```python
from build123d import *

# Parameters (mm, degrees)
SKETCH1_R                                           = 60.625
SKETCH1_R_2                                         = 45
BOSS_EXTRUDE1_DEPTH                                 = 4
SKETCH2_R                                           = 49
SKETCH2_R_2                                         = 45
BOSS_EXTRUDE2_DEPTH                                 = 52
SKETCH4_W                                           = 13.25
SKETCH4_H                                           = 8
SKETCH4_W_2                                         = 8
SKETCH4_H_2                                         = 38
BOSS_EXTRUDE4_DEPTH                                 = 13
BOSS_EXTRUDE5_DEPTH                                 = 4
SKETCH7_R                                           = 1.3
CUT_EXTRUDE4_DEPTH                                  = 7.2
SKETCH9_W                                           = 10
SKETCH9_H                                           = 24
CUT_EXTRUDE7_DEPTH                                  = 8
CUT_EXTRUDE8_REACH                                  = 111.625
SKETCH11_R                                          = 5
CUT_EXTRUDE9_DEPTH                                  = 5.0000001
CSK_FOR_M3_COUNTERSUNK_FLAT_HEAD_SCREW1_D           = 3.4
CSK_FOR_M3_COUNTERSUNK_FLAT_HEAD_SCREW1_DEPTH       = 4
CSK_FOR_M3_COUNTERSUNK_FLAT_HEAD_SCREW1_CSINK_D     = 6.3
CSK_FOR_M3_COUNTERSUNK_FLAT_HEAD_SCREW1_CSINK_ANGLE = 90
SKETCH18_W                                          = 98
SKETCH18_H                                          = 7
CUT_EXTRUDE10_DEPTH                                 = 61.625
CUT_EXTRUDE10_DEPTH_BACK                            = 61.625


with BuildPart() as part:
    # Sketch1 → Boss-Extrude1 (new body)
    with BuildSketch(Plane(origin=(0, 0, 0), x_dir=(1, 0, 0), z_dir=(0, 1, 0))):
        Circle(SKETCH1_R)
        Circle(SKETCH1_R_2, mode=Mode.SUBTRACT)
    extrude(amount=BOSS_EXTRUDE1_DEPTH)

    # Sketch2 → Boss-Extrude2 (add)
    with BuildSketch(Plane(origin=(0, 4, 0), x_dir=(1, 0, 0), z_dir=(0, 1, 0))):
        Circle(SKETCH2_R)
        Circle(SKETCH2_R_2, mode=Mode.SUBTRACT)
    extrude(amount=BOSS_EXTRUDE2_DEPTH)

    # Sketch4 → Boss-Extrude4 (add, symmetric)
    with BuildSketch(Plane.XY):
        with Locations((-38.375, 34)):
            Rectangle(SKETCH4_W, SKETCH4_H)
        Polygon((-31.75, 30), (-45, 30), (-45, 16.75), align=None)
        with Locations((15.25, 19)):
            Rectangle(SKETCH4_W_2, SKETCH4_H_2)
    extrude(amount=BOSS_EXTRUDE4_DEPTH, both=True)

    # Sketch5 → Boss-Extrude5 (add)
    with BuildSketch(Plane.XZ):
        with BuildLine():
            Line((11.25, 13), (29.067400866, 34.352382842))
            ThreePointArc((29.067400866, 34.352382842), (45, 0), (29.067400866, -34.352382842))
            Line((29.067400866, -34.352382842), (11.25, -13))
            Line((11.25, -13), (11.25, 13))
        make_face()
    extrude(amount=-BOSS_EXTRUDE5_DEPTH)

    # Sketch7 → Cut-Extrude4 (cut)
    with BuildSketch(Plane(origin=(0, 38, 0), x_dir=(1, 0, 0), z_dir=(0, 1, 0))):
        with Locations((-34.25, 5)):
            Circle(SKETCH7_R)
        with Locations((-34.25, -5)):
            Circle(SKETCH7_R)
        with Locations((13.75, 5)):
            Circle(SKETCH7_R)
        with Locations((13.75, -5)):
            Circle(SKETCH7_R)
    extrude(amount=-CUT_EXTRUDE4_DEPTH, mode=Mode.SUBTRACT)

    # Sketch9 → Cut-Extrude7 (cut)
    with BuildSketch(Plane.ZY.offset(-11.25)):
        with Locations((0, 17)):
            Rectangle(SKETCH9_W, SKETCH9_H)
    extrude(amount=-CUT_EXTRUDE7_DEPTH, mode=Mode.SUBTRACT)

    # Sketch11 → Cut-Extrude8 (cut, up to next)
    with BuildSketch(Plane(origin=(49, 0, 0), x_dir=(0, 0, -1), z_dir=(1, 0, 0)), mode=Mode.PRIVATE) as cut_extrude8_sk1:
        with Locations((0, 14)):
            Circle(SKETCH11_R)
    cut_extrude8_tool1 = extrude(cut_extrude8_sk1.sketch, amount=-CUT_EXTRUDE8_REACH, mode=Mode.PRIVATE) & part.part
    add(cut_extrude8_tool1.solids().sort_by_distance((49, 14, 0))[0], mode=Mode.SUBTRACT)

    # Sketch12 → Cut-Extrude9 (cut, through all)
    with BuildSketch(Plane(origin=(0, 4, 0), x_dir=(1, 0, 0), z_dir=(0, 1, 0))):
        with BuildLine():
            Line((29.479537487, 22.359715328), (27.25, 19.687836398))
            Line((27.25, 19.687836398), (27.25, -19.687836398))
            Line((27.25, -19.687836398), (29.479537487, -22.359715328))
            ThreePointArc((29.479537487, -22.359715328), (37, 0), (29.479537487, 22.359715328))
        make_face()
        Polygon((27.25, -19.687836398), (27.25, 19.687836398), (24.25, 16.092634774), (24.25, -16.092634774), align=None)
    extrude(amount=-CUT_EXTRUDE9_DEPTH, mode=Mode.SUBTRACT)

    # CSK for M3 Countersunk Flat Head Screw1
    with Locations(Plane(origin=(0, 4, 0), x_dir=(1, 0, 0), z_dir=(0, 1, 0))):
        with Locations((-38.890872965, 38.890872965), (-38.890872965, -38.890872965), (38.890872965, -38.890872965), (38.890872965, 38.890872965)):
            CounterSinkHole(CSK_FOR_M3_COUNTERSUNK_FLAT_HEAD_SCREW1_D / 2, CSK_FOR_M3_COUNTERSUNK_FLAT_HEAD_SCREW1_CSINK_D / 2, depth=CSK_FOR_M3_COUNTERSUNK_FLAT_HEAD_SCREW1_DEPTH, counter_sink_angle=CSK_FOR_M3_COUNTERSUNK_FLAT_HEAD_SCREW1_CSINK_ANGLE)

    # Sketch18 → Cut-Extrude10 (cut, two sides)
    with BuildSketch(Plane.XY) as cut_extrude10_sk:
        with Locations((0, 56)):
            Rectangle(SKETCH18_W, SKETCH18_H)
    extrude(amount=CUT_EXTRUDE10_DEPTH, mode=Mode.SUBTRACT)
    extrude(cut_extrude10_sk.sketch, amount=-CUT_EXTRUDE10_DEPTH_BACK, mode=Mode.SUBTRACT)


solid = part.part
```
Model file for the job. Use its own axes, mm. A direction names the side the tool comes from. Give positions to 0.01 mm unless a question says otherwise; leave off trailing zeros. Loops run counter-clockwise (first coordinate to the right, second up) from the corner with the lowest first, then second, coordinate; pieces in that order, holes last. Notation, with made-up numbers: M 12,77 L 61,77 A29 ccw 61,107 Z; hole C 19,73 d7. An arc over 180 degrees is marked long. Use one line per item in the form item = value.
Item 1: Slice it at C-C on y = 35. List the corners of the cut face in (x, z), and give its area (3 significant figures).
Filled in:
outline = C 0,0 d98; M 11.25,-13 L 19.25,-13 L 19.25,13 L 11.25,13 Z; hole M -43.08,-13 A45 ccw long -43.08,13 L -31.75,13 L -31.75,-13 Z; hole C -34.25,-5 d2.6; hole C -34.25,5 d2.6; hole C 13.75,-5 d2.6; hole C 13.75,5 d2.6
area = 1,700 mm^2
Item 2: Two-plate mould, pull along Z, no slides. Class faces 1 (the flat face through (11.25, 19, 6)), 2 (the flat face through (-38, 38, 0)), 3 (the cylindrical face through (26.34, 27.91, -41.32)): released by +Z, released by -Z, zero draft, split by the parting line, or undercut.
Filled in:
face_1 = undercut
face_2 = undercut
face_3 = split by the parting line
Item 3: Slice it at B-B on z = 0. Give the number of separate pieces and of enclosed holes in the cut face, and give its area (3 significant figures).
Filled in:
separate_pieces = 5
enclosed_holes = 0
area = 831 mm^2
Item 4: Slice it at A-A on y = 6.5. List the corners of the cut face in (x, z).
Filled in:
outline = C 0,0 d98; M 11.25,-13 L 19.25,-13 L 19.25,-5 L 11.25,-5 Z; M 11.25,5 L 19.25,5 L 19.25,13 L 11.25,13 Z; hole C 0,0 d90
Item 5: Slice it at D-D on x = -22.5. List the corners of the cut face in (y, z).
Filled in:
outline = M 0,-56.3 L 4,-56.3 L 4,-43.53 L 52.5,-43.53 L 52.5,-38.97 L 0,-38.97 Z; M 0,38.97 L 52.5,38.97 L 52.5,43.53 L 4,43.53 L 4,56.3 L 0,56.3 Z
Item 6: Flat gauge pins, fed straight in: pin 1 Ø10 at (x, z) = (25, -1.5) entering from +Y; pin 2 Ø2 at (x, y) = (-1.5, 47) entering from -Z; pin 3 Ø3 at (x, z) = (13.5, 4.5) entering from +Y; pin 4 Ø5 at (x, z) = (-24.5, -47.5) entering from -Y. Where does each tip first touch, or does it go through?
Filled in:
pin_1 = 4
pin_2 = -49
pin_3 = 38
pin_4 = 0
Item 7: Drill centre lines: L1, parallel to X at y = 3.5, z = 1.5 (3 decimals); L2, parallel to Z at x = -34.25, y = 34; L3, parallel to Z at x = 19, y = 23.5. Where is each one in solid material? Low to high.
Filled in:
L1 = -60.606 to -44.975, 11.25 to 24.25, 36.97 to 60.606
L2 = -35.04 to -29.19, -13 to -6.3, -3.7 to 3.7, 6.3 to 13, 29.19 to 35.04
L3 = -45.17 to -40.79, -13 to -5, 5 to 13, 40.79 to 45.17
Item 8: Which spindle directions (+Z, -Z, +X, -X, +Y, -Y) get a long thin tool onto all of the face, cutting with end or side? Do faces 4 (the flat face through (15, 21, 13)), 5 (the flat face through (15, 29, 0)), 6 (the flat face through (-39, 31, 13)). Say none if no direction does.
Filled in:
face_4 = +Y
face_5 = none
face_6 = +Y, -Y
